from build123d import *

# Parameters (mm, degrees)
SKETCH037_W     = 72.5
SKETCH037_H     = 55
PAD018_DEPTH    = 60
SKETCH038_W     = 67.9
SKETCH038_H     = 50.4
POCKET013_DEPTH = 60.001
SKETCH039_W     = 67.9
SKETCH039_H     = 4
PAD019_DEPTH    = 50.4
SKETCH040_R     = 2.2
HOLE006_DEPTH   = 25
SKETCH041_W     = 28
SKETCH041_H     = 43
POCKET014_DEPTH = 4
SKETCH042_W     = 33
SKETCH042_H     = 50.4
SKETCH042_W_2   = 28
SKETCH042_H_2   = 43
PAD020_DEPTH    = 40
SKETCH043_W     = 20
SKETCH043_H     = 2
PAD021_DEPTH    = 43


with BuildPart() as part:
    # Sketch037 → Pad018 (new body)
    with BuildSketch(Plane.YZ.offset(120)):
        with Locations((1.26, 27.5)):
            Rectangle(SKETCH037_W, SKETCH037_H)
    extrude(amount=PAD018_DEPTH)

    # Sketch038 (on Face5 of Pad018) → Pocket013 (cut, through all)
    with BuildSketch(Plane(origin=(120, 0, 0), x_dir=(0, 1, 0), z_dir=(-1, 0, 0))):
        with Locations((1.25, -27.5)):
            Rectangle(SKETCH038_W, SKETCH038_H)
    extrude(amount=-POCKET013_DEPTH, mode=Mode.SUBTRACT)

    # Sketch039 (on Face8 of Pocket013) → Pad019 (join)
    with BuildSketch(Plane(origin=(0, 0, 2.3), x_dir=(0, -1, 0), z_dir=(0, 0, 1))):
        with Locations((-1.25, 130)):
            Rectangle(SKETCH039_W, SKETCH039_H)
    extrude(amount=PAD019_DEPTH)

    # Sketch040 (on Face16 of Pad019) → Hole006 (cut)
    with BuildSketch(Plane.YZ.offset(132)):
        with Locations((-25.99, 42.5)):
            Circle(SKETCH040_R)
        with Locations((-23, 9)):
            Circle(SKETCH040_R)
        with Locations((23, 9)):
            Circle(SKETCH040_R)
    extrude(amount=-HOLE006_DEPTH, mode=Mode.SUBTRACT)

    # Sketch041 (on Face16 of Hole006) → Pocket014 (cut)
    with BuildSketch(Plane.YZ.offset(132)):
        with Locations((0, 27.5)):
            Rectangle(SKETCH041_W, SKETCH041_H)
    extrude(amount=-POCKET014_DEPTH, mode=Mode.SUBTRACT)

    # Sketch042 (on Face16 of Pocket014) → Pad020 (join)
    with BuildSketch(Plane.YZ.offset(132)):
        with Locations((0, 27.5)):
            Rectangle(SKETCH042_W, SKETCH042_H)
        with Locations((0, 27.5)):
            Rectangle(SKETCH042_W_2, SKETCH042_H_2, mode=Mode.SUBTRACT)
    extrude(amount=PAD020_DEPTH)

    # Sketch043 (on Face29 of Pad020) → Pad021 (join)
    with BuildSketch(Plane(origin=(0, 0, 6), x_dir=(0, -1, 0), z_dir=(0, 0, 1))):
        with Locations((-4, 168.5)):
            Rectangle(SKETCH043_W, SKETCH043_H)
        with Locations((4, 156.75)):
            Rectangle(SKETCH043_W, SKETCH043_H)
        with Locations((-4, 145)):
            Rectangle(SKETCH043_W, SKETCH043_H)
    extrude(amount=PAD021_DEPTH)


solid = part.part
Read the model definition and answer for the solid it produces. Units are mm, in the model's axes. A direction names the side the tool comes from. Round coordinates to 2 decimals unless told otherwise and drop trailing zeros. Write each loop counter-clockwise with the first axis right and the second up, starting at its lowest first coordinate (ties: lowest second). Pieces come first, ordered by that corner, then holes. Notation, with made-up numbers: (-30.75, 70.5) - (3.25, 70.5) arc R24 cw to (3.25, 91.5) - close; hole circle Ø6 at (-21, 19). An arc over 180 degrees is marked (long way). One line per question, with ' | ' between items. Start each with the question number.
1. Section C-C (y = 9.5) is taken. Determine the outline of the cut face in (x, z).
2. For a pull along Y with two mould halves and no side action, classify faces 6 (the face through (150, -34.99, 27)), 7 (the face through (130.028, -26.467, 40.352)), 8 (the face through (180, -2, 1)) as +Y half, -Y half, draft (parallel to the pull), parting line (faces both ways), or undercut.
3. Section B-B (x = 171) is taken. Determine the outline of the cut face in (y, z), and give its area (3 significant figures).
4. Section D-D (y = 23) is taken. Determine the outline of the cut face in (x, z), and give its area (3 significant figures).
5. Find the intervals of material crossed by probe 1 along Y at (x, z) = (155, 38); probe 2 along X at (y, z) = (3, 16); probe 3 along Y at (x, z) = (143, 52.5), in increasing order. Write a range as [from, to].
6. For faces 1 (the face through (130.03, -20.9, 9.66)), 2 (the face through (124, 1, 2.3)), 3 (the face through (177, 1, 52.7)), 4 (the face through (150, 1, 0)), 5 (the face through (157.75, -4, 27)), determine the directions among +Z, -Z, +X, -X, +Y, -Y from which every point of the face is accessible in a straight line to the end or side of a thin tool.
7. Each of these flat-tipped pins is pushed along its axis until it touches: pin 1 (5 mm diameter, centred on y = 23, z = 9, fed in from -X); pin 2 (5 mm diameter, centred on y = -25.99, z = 42.5, fed in from +X); pin 3 (6 mm diameter, centred on y = 5.5, z = 36.5, fed in from +X). Where does it stop, or does it pass through?
Filled in:
1) outline: (120, 0) - (180, 0) - (180, 2.3) - (172, 2.3) - (172, 6) - (169.5, 6) - (169.5, 49) - (172, 49) - (172, 52.7) - (180, 52.7) - (180, 55) - (120, 55) - (120, 52.7) - (128, 52.7) - (128, 49) - (144, 49) - (144, 6) - (128, 6) - (128, 2.3) - (120, 2.3) - close; hole (146, 6) - (167.5, 6) - (167.5, 49) - (146, 49) - close
2) face 6: -Y half | face 7: undercut | face 8: draft
3) outline: (-34.99, 0) - (37.51, 0) - (37.51, 55) - (-34.99, 55) - close; hole (-32.7, 2.3) - (-16.5, 2.3) - (-16.5, 52.7) - (-32.7, 52.7) - close; hole (-14, 6) - (14, 6) - (14, 49) - (-14, 49) - close; hole (16.5, 2.3) - (35.2, 2.3) - (35.2, 52.7) - (16.5, 52.7) - close | area: 1,020 mm²
4) outline: (120, 0) - (180, 0) - (180, 2.3) - (132, 2.3) - (132, 6.8) - (128, 6.8) - (128, 2.3) - (120, 2.3) - close; (120, 52.7) - (128, 52.7) - (128, 11.2) - (132, 11.2) - (132, 52.7) - (180, 52.7) - (180, 55) - (120, 55) - close | area: 460 mm²
5) probe 1: [-34.99, -32.7], [-16.5, -14], [14, 16.5], [35.2, 37.51] | probe 2: [144, 146], [155.75, 157.75], [167.5, 169.5] | probe 3: [-34.99, -32.7], [-16.5, 16.5], [35.2, 37.51]
6) face 1: +X, -X | face 2: -X | face 3: +X | face 4: -Z, +X, -X, +Y, -Y | face 5: none
7) pin 1: x = 128 | pin 2: x = 132 | pin 3: x = 169.5
